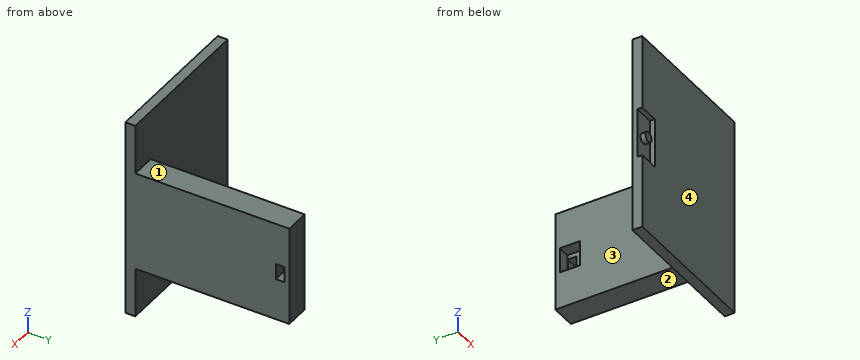
from build123d import *

# Parameters (mm, degrees)
ESQUISSE2_W             = 150
ESQUISSE2_H             = 200
BOSS_EXTRU_6_DEPTH      = 10
ESQUISSE4_W             = 25
ESQUISSE4_H             = 100
BOSS_EXTRU_7_DEPTH      = 160
ESQUISSE8_W             = 24.4
ESQUISSE8_H             = 20.028297961
ENL_V_MAT_EXTRU_1_DEPTH = 12.2
ESQUISSE9_W             = 12
ESQUISSE9_H             = 5
ENL_V_MAT_EXTRU_2_DEPTH = 42.2
ESQUISSE11_W            = 16
ESQUISSE11_H            = 8.51414898
ENL_V_MAT_EXTRU_3_DEPTH = 42.2
ENL_V_MAT_EXTRU_6_DEPTH = 12.2
ESQUISSE13_W            = 25
ESQUISSE13_H            = 100
BOSS_EXTRU_8_DEPTH      = 5
ESQUISSE14_W            = 25.4
ESQUISSE14_H            = 0.5
ENL_V_MAT_EXTRU_7_DEPTH = 12.2
ESQUISSE19_W            = 50
ESQUISSE19_H            = 5
ENL_V_MAT_EXTRU_8_DEPTH = 150
BOSS_EXTRU_9_DEPTH      = 42
BOSS_EXTRU_9_DEPTH_BACK = 75
ESQUISSE21_W            = 50
ESQUISSE21_H            = 5
ESQUISSE22_R            = 5
BOSS_EXTRU_10_DEPTH     = 6


with BuildPart() as part:
    # Esquisse2 → Boss.-Extru.6 (new body)
    with BuildSketch(Plane(origin=(0, 0, 0), x_dir=(1, 0, 0), z_dir=(0, 1, 0))):
        with Locations((-20.308131119, 81.7)):
            Rectangle(ESQUISSE2_W, ESQUISSE2_H)
    extrude(amount=BOSS_EXTRU_6_DEPTH)

    # Esquisse4 → Boss.-Extru.7 (add)
    with BuildSketch(Plane(origin=(0, 0, 0), x_dir=(1, 0, 0), z_dir=(0, 1, 0))):
        with Locations((42.191868881, 81.7)):
            Rectangle(ESQUISSE4_W, ESQUISSE4_H)
    extrude(amount=BOSS_EXTRU_7_DEPTH)

    # Esquisse8 → Enlèv. mat.-Extru.1 (cut)
    with BuildSketch(Plane.ZY.offset(-29.691868881)):
        with Locations((-81.7, 149.985851019)):
            Rectangle(ESQUISSE8_W, ESQUISSE8_H)
    extrude(amount=-ENL_V_MAT_EXTRU_1_DEPTH, mode=Mode.SUBTRACT)

    # Esquisse9 → Enlèv. mat.-Extru.2 (cut)
    with BuildSketch(Plane.ZY.offset(-41.891868881)):
        with Locations((-81.7, 155.98585102)):
            Rectangle(ESQUISSE9_W, ESQUISSE9_H)
    extrude(amount=-ENL_V_MAT_EXTRU_2_DEPTH, mode=Mode.SUBTRACT)

    # Esquisse11 → Enlèv. mat.-Extru.3 (cut)
    with BuildSketch(Plane.ZY.offset(-41.891868881)):
        with Locations((-81.7, 155.74292551)):
            Rectangle(ESQUISSE11_W, ESQUISSE11_H)
    extrude(amount=-ENL_V_MAT_EXTRU_3_DEPTH, mode=Mode.SUBTRACT)

    # Esquisse12 → Enlèv. mat.-Extru.6 (cut)
    with BuildSketch(Plane.ZY.offset(-29.691868881)):
        Polygon((-94.4, 160), (-94.4, 139.97), (-93.9, 139.971702039), (-93.9, 160), align=None)
        Polygon((-69, 139.97), (-69, 160), (-69.5, 160), (-69.5, 139.971702039), align=None)
    extrude(amount=-ENL_V_MAT_EXTRU_6_DEPTH, mode=Mode.SUBTRACT)

    # Esquisse13 → Boss.-Extru.8 (add)
    with BuildSketch(Plane(origin=(0, 160, 0), x_dir=(1, 0, 0), z_dir=(0, 1, 0))):
        with Locations((42.191868881, 81.7)):
            Rectangle(ESQUISSE13_W, ESQUISSE13_H)
    extrude(amount=BOSS_EXTRU_8_DEPTH)

    # Esquisse14 → Enlèv. mat.-Extru.7 (cut)
    with BuildSketch(Plane.ZY.offset(-29.691868881)):
        with Locations((-81.7, 160.25)):
            Rectangle(ESQUISSE14_W, ESQUISSE14_H)
    extrude(amount=-ENL_V_MAT_EXTRU_7_DEPTH, mode=Mode.SUBTRACT)

    # Esquisse19 → Enlèv. mat.-Extru.8 (cut)
    with BuildSketch(Plane.ZY.offset(-41.891868881)):
        with Locations((-81.7, 2.5)):
            Rectangle(ESQUISSE19_W, ESQUISSE19_H)
    extrude(amount=ENL_V_MAT_EXTRU_8_DEPTH, mode=Mode.SUBTRACT)

    # Esquisse21 → Boss.-Extru.9 (add, two sides: drawn at the far end of the back side and taken through both)
    with BuildSketch(Plane(origin=(0, 0, 0), x_dir=(0, 0, -1), z_dir=(1, 0, 0)).offset(-BOSS_EXTRU_9_DEPTH_BACK)):
        with Locations((81.7, 2.5)):
            Rectangle(ESQUISSE21_W, ESQUISSE21_H)
    extrude(amount=BOSS_EXTRU_9_DEPTH + BOSS_EXTRU_9_DEPTH_BACK)

    # Esquisse22 → Boss.-Extru.10 (add)
    with BuildSketch(Plane(origin=(0, 0, 0), x_dir=(1, 0, 0), z_dir=(0, 1, 0))):
        with Locations(Location((-85.154065559, 81.7, 0), (0, 0, 90))):
            Circle(ESQUISSE22_R)
    extrude(amount=BOSS_EXTRU_10_DEPTH)


solid = part.part
Work out the finished part from the listing and answer in its coordinate system (mm). Face numbers are marked on the shaded views. A direction names the side the tool comes from. Give positions to 0.01 mm unless a question says otherwise; leave off trailing zeros. Order: outer loops, then holes, each group sorted by start corner. A loop starts at its lowest first (then second) coordinate and runs counter-clockwise, first axis right, second up. Notation, with made-up numbers: M -36.5,1.25 L -21.5,1.25 A30 ccw -21.5,32.25 Z; hole C 58,47.5 d5. An arc over 180 degrees is marked long. Return JSON: item names as keys, results as strings.
Q1. Find section C-C, the plane z = -60. Write down the section's boundary in (x, y), and give its area (3 significant figures).
Answer below:
{"outline": "M -95.31,5 L -75,5 L -75,0 L 54.69,0 L 54.69,165 L 29.69,165 L 29.69,10 L -95.31,10 Z", "area": "5,270 mm^2"}
Q2. Which of the six approach directions +Z, -Z, +X, -X, +Y, -Y give full straight-line access (tool end or side, diameter ignored) to the marked faces 1, 2, 3 and 4?
Answer below:
{"face 1": "+Z, +X, -X, +Y", "face 2": "-Z, +X, -X, +Y", "face 3": "+Z, -Z, -X, +Y", "face 4": "+Z, -Z, +X, -X, -Y"}
Q3. Find the intervals of material crossed by line 1 along X through (y, z) = (37, -113); line 2 along Y through (x, z) = (-48, -162); line 3 along Z through (x, y) = (45.5, 151), in increasing order. Write a range as [from, to].
Answer below:
{"line 1": "x = [29.69, 54.69]", "line 2": "y = [0, 10]", "line 3": "z = [-131.7, -31.7]"}
Q4. Find section B-B, the plane z = -81.7. Write down the section's boundary in (x, y).
Answer below:
{"outline": "M -95.31,5 L -90.15,5 L -90.15,0 L -80.15,0 L -80.15,5 L -75,5 L -75,0 L 54.69,0 L 54.69,151.49 L 41.89,151.49 L 41.89,139.97 L 29.69,139.97 L 29.69,10 L -95.31,10 Z; M 29.69,160.5 L 41.89,160.5 L 41.89,160 L 54.69,160 L 54.69,165 L 29.69,165 Z"}
Q5. Each of these flat-tipped pins is pushed along its axis until it touches: pin 1 (3 mm diameter, centred on x = 33.5, y = 21.5, fed in from +Z); pin 2 (13.5 mm diameter, centred on x = 36, y = 148, fed in from -Z); pin 3 (6 mm diameter, centred on y = 148, z = -81.5, fed in from -X). Where does it stop, or does it pass through?
Answer below:
{"pin 1": "stops at z = -31.7", "pin 2": "stops at z = -131.7", "pin 3": "stops at x = 41.89"}
Q6. Find section A-A, the plane y = 154.5. Write down the section's boundary in (x, z), and give its area (3 significant figures).
Answer below:
{"outline": "M 29.69,-131.7 L 54.69,-131.7 L 54.69,-89.7 L 41.89,-89.7 L 41.89,-94.4 L 29.69,-94.4 Z; M 29.69,-69 L 41.89,-69 L 41.89,-73.7 L 54.69,-73.7 L 54.69,-31.7 L 29.69,-31.7 Z", "area": "1,990 mm^2"}
Q7. Find section D-D, the plane x = -49.5. Write down the section's boundary in (y, z).
Answer below:
{"outline": "M 0,-181.7 L 10,-181.7 L 10,18.3 L 0,18.3 Z"}
